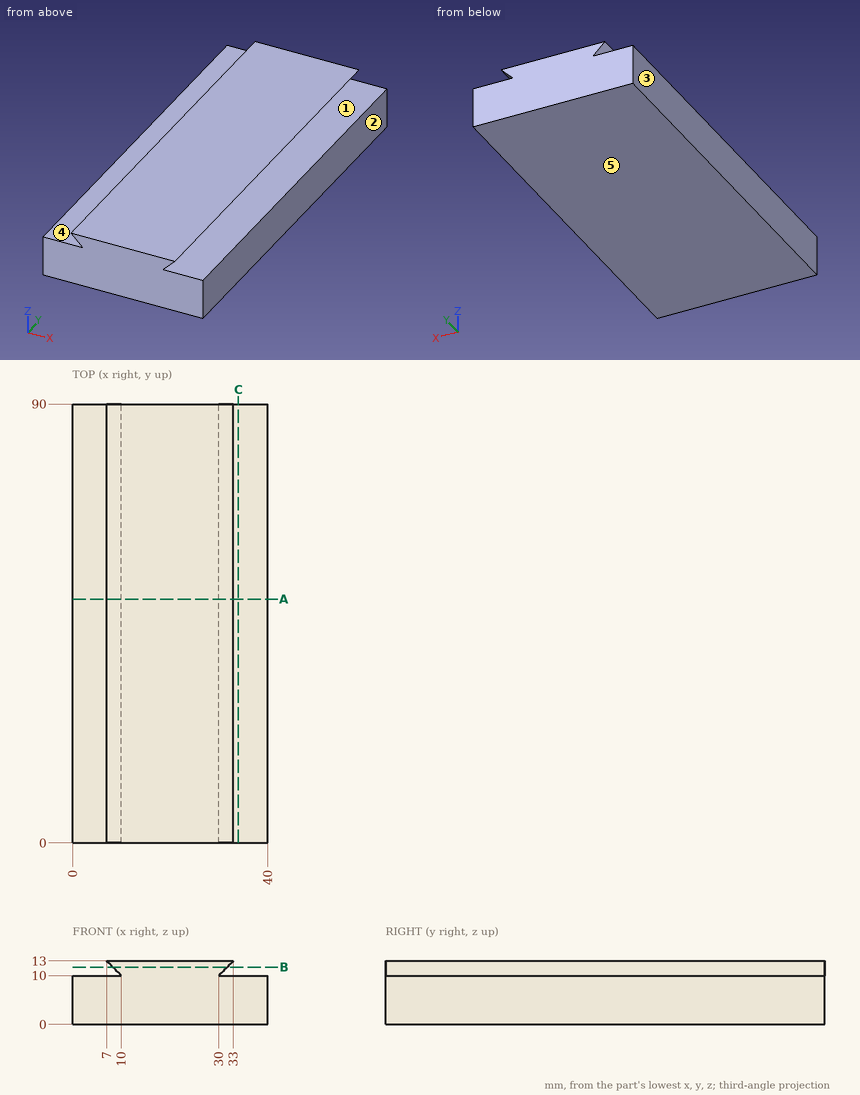
Input: dimensioned drawing with shaded views. Units: mm. Origin: part minimum x, y, z. A direction names the side the tool comes from. Coordinates: 2 decimals unless noted, no trailing zeros. Write each loop counter-clockwise with the first axis right and the second up, starting at its lowest first coordinate (ties: lowest second). Pieces come first, ordered by that corner, then holes. Notation, with made-up numbers: M 12,-35.75 L 58,-35.75 A23 cw 58,-17.75 Z; hole C -17.5,14.5 d6. An arc over 180 degrees is marked long. Answer as CSV lines item,"result". Start each with the question number.
Q1. Cut plane C-C on x = 34. Return the cut outline in (y, z).
Q2. Line query: line 1 (Z direction, x = 38.5, y = 29); line 2 (Z direction, x = 9, y = 63.5). Output: solid intervals per line, ascending. Write a range as from..to.
Q3. Reachability of the marked faces 1 and 2 from +Z, -Z, +X, -X, +Y, -Y: full face, straight path, thin tool, end or side. Return the list, or none.
Q4. Cut plane A-A on y = 50. Return the cut outline in (x, z).
Q5. Mould query, pull axis Z, two halves, no side actions, for the marked faces 3, 4 and 5. Classes: released by +Z, released by -Z, zero draft, split by the parting line, or undercut.
Q6. Cut plane B-B on z = 11.75. Return the cut outline in (x, y).
Q7. Pin query (flat end, axial travel): P1, Ø2, axis at y = 56.5, z = 5.5, coming from the -X side; P2, Ø5, axis at x = 3, y = 37.5, coming from the +Z side. Return the tip coordinate at first contact, or that it passes through.
Findings below:
1,outline,"M 0,0 L 90,0 L 90,10 L 0,10 Z"
2,line 1,"z = 0..10"
2,line 2,"z = 0..10, 11..13"
3,face 1,"+X, +Y, -Y"
3,face 2,"+Z, -Z, +X, +Y, -Y"
4,outline,"M 0,0 L 40,0 L 40,10 L 30,10 L 33,13 L 7,13 L 10,10 L 0,10 Z"
5,face 3,"zero draft"
5,face 4,"undercut"
5,face 5,"released by -Z"
6,outline,"M 8.25,0 L 31.75,0 L 31.75,90 L 8.25,90 Z"
7,P1,"stops at x = 0"
7,P2,"stops at z = 10"
